Here's the drawing with two shaded views (mm, measured from the low corner). I have some questions. A direction names the side the tool comes from. Give positions to 0.01 mm unless a question says otherwise; leave off trailing zeros. Write each loop counter-clockwise with the first axis right and the second up, starting at its lowest first coordinate (ties: lowest second). Pieces come first, ordered by that corner, then holes. Notation, with made-up numbers: (4, 89.5) -> (23, 89.5) arc R14 ccw to (23, 114.5) -> close; hole circle Ø1 at (68, 66.5). An arc over 180 degrees is marked (long way). One line per question, with ' | ' between items.
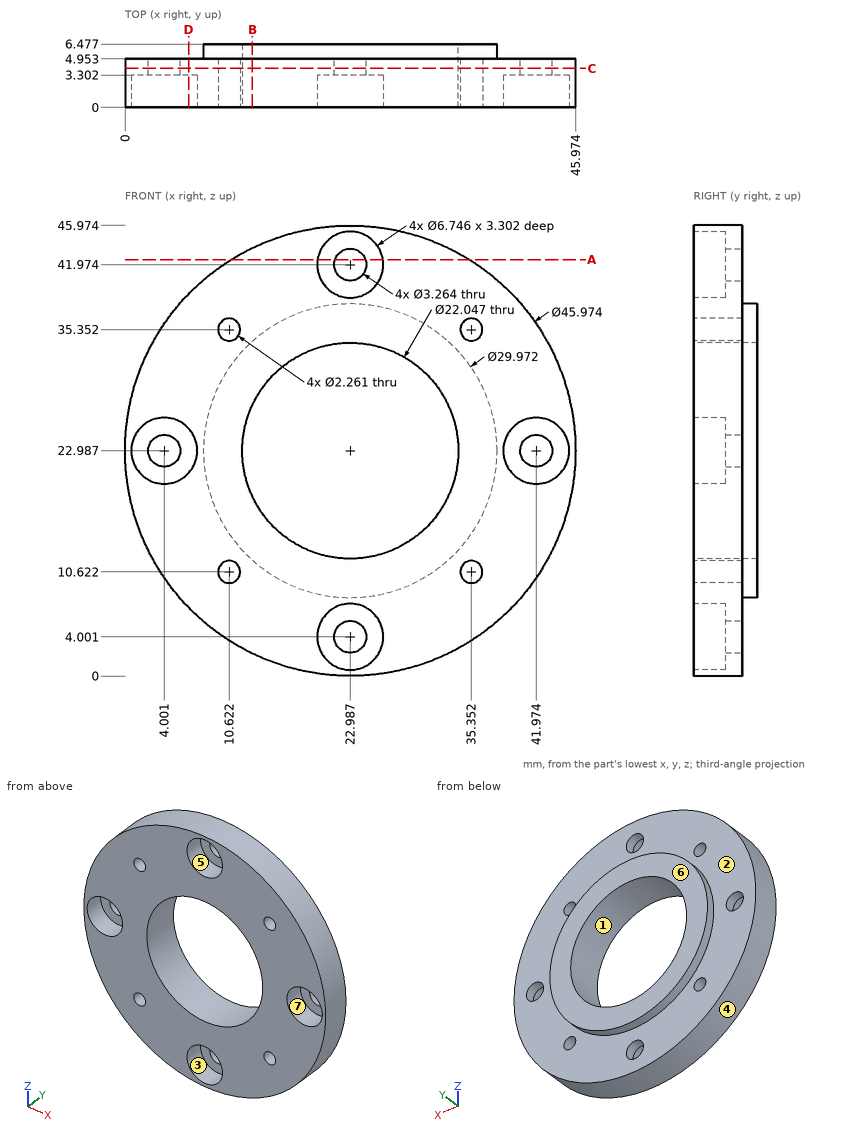
Q1. Imagine slicing it at D-D on x = 6.5. Please give me the cut outline in (y, z) (1 decimal).
Answer below:
outline: (0, 7) -> (5, 7) -> (5, 39) -> (0, 39) -> (0, 25.3) -> (3.3, 25.3) -> (3.3, 20.7) -> (0, 20.7) -> close
Q2. On a 3-axis mill with a long thin cutter (end or side, diameter ignored), from which of +Z, -Z, +X, -X, +Y, -Y can I reach the whole of each face in a straight line? I mean the marked faces 1, 2 and 3. Say none if no direction works.
Answer below:
face 1: +Y, -Y | face 2: +Y | face 3: -Y
Q3. Will these pins go through, and if not, where does the flat tip stop? pin 1 (4 mm diameter, centred on x = 22.99, z = 41.97, fed in from +Y); pin 2 (2 mm diameter, centred on x = 21.5, z = 42.5, fed in from -Y); pin 3 (2 mm diameter, centred on y = 3, z = 15.5, fed in from -X) (1 decimal).
Answer below:
pin 1: stops at y = 4.95 | pin 2: stops at y = 3.3 | pin 3: stops at x = 0.9
Q4. If I drill on line 1 along X through (y, z) = (1, 26) (1 decimal); line 2 along Z through (x, y) = (35.5, 3.5) (1 decimal); line 3 along Z through (x, y) = (22.5, 0.5) (1 decimal), over which ranges is the centre line in solid material (lowest first)?
Answer below:
line 1: x = 0.2 to 2.5, 5.5 to 12.4, 33.6 to 40.5, 43.5 to 45.8 | line 2: z = 3.7 to 9.5, 11.7 to 34.2, 36.5 to 42.3 | line 3: z = 0 to 0.7, 7.3 to 12, 34 to 38.6, 45.3 to 46
Q5. If we mould it in two halves opening along X, with no side actions, what happens to the marked faces 4, 5, 6 and 7? For each: +X half, -X half, draft (parallel to the pull), parting line (faces both ways), or undercut.
Answer below:
face 4: parting line | face 5: undercut | face 6: draft | face 7: undercut
Q6. Imagine slicing it at A-A on z = 42.5. Please give me the cut outline in (x, y) (1 decimal).
Answer below:
outline: (10.8, 0) -> (19.7, 0) -> (19.7, 3.3) -> (21.4, 3.3) -> (21.4, 5) -> (10.8, 5) -> close; (24.5, 3.3) -> (26.3, 3.3) -> (26.3, 0) -> (35.1, 0) -> (35.1, 5) -> (24.5, 5) -> close
Q7. Imagine slicing it at B-B on x = 13. Please give me the cut outline in (y, z), and give its area (3 significant figures).
Answer below:
outline: (0, 2.28) -> (4.95, 2.28) -> (4.95, 11.81) -> (6.48, 11.81) -> (6.48, 18.32) -> (0, 18.32) -> close; (0, 27.65) -> (6.48, 27.65) -> (6.48, 34.16) -> (4.95, 34.16) -> (4.95, 43.69) -> (0, 43.69) -> close | area: 179 mm^2
Q8. Imagine slicing it at C-C on y = 4. Count the separate pieces of the cut face and the enclosed holes in it, and give its area (3 significant figures).
Answer below:
separate pieces: 1 | enclosed holes: 9 | area: 1,230 mm^2
